from build123d import *

# Parameters (mm, degrees)
F0_R     = 5
F1_DEPTH = 2
F2_DEPTH = 2
F3_DEPTH = 2
F4_DEPTH = 2


with BuildPart() as f1:
    # F0 (on Top) → F1 (new body)
    with BuildSketch(Plane.XY):
        Circle(F0_R)
        with BuildLine():
            ThreePointArc((3.8729833462, 1), (3.9681187851, 0.5040171699), (4, 0))
            ThreePointArc((4, 0), (3.9681187851, -0.5040171699), (3.8729833462, -1))
            ThreePointArc((3.8729833462, -1), (3.5772466103, -1.789778391), (3.1224989992, -2.5))
            ThreePointArc((3.1224989992, -2.5), (2.9455449899, -2.7062455011), (2.7549954628, -2.9))
            ThreePointArc((2.7549954628, -2.9), (0, -4), (-2.7549954628, -2.9))
            ThreePointArc((-2.7549954628, -2.9), (-2.9455449899, -2.7062455011), (-3.1224989992, -2.5))
            ThreePointArc((-3.1224989992, -2.5), (-3.5772466103, -1.789778391), (-3.8729833462, -1))
            ThreePointArc((-3.8729833462, -1), (-4, 0), (-3.8729833462, 1))
            ThreePointArc((-3.8729833462, 1), (-3.5772466103, 1.789778391), (-3.1224989992, 2.5))
            ThreePointArc((-3.1224989992, 2.5), (-2.9455449899, 2.7062455011), (-2.7549954628, 2.9))
            ThreePointArc((-2.7549954628, 2.9), (0, 4), (2.7549954628, 2.9))
            ThreePointArc((2.7549954628, 2.9), (2.9455449899, 2.7062455011), (3.1224989992, 2.5))
            ThreePointArc((3.1224989992, 2.5), (3.5772466103, 1.789778391), (3.8729833462, 1))
        make_face(mode=Mode.SUBTRACT)
    extrude(amount=F1_DEPTH)

    # F0 (on Top) → F2 (join)
    with BuildSketch(Plane.XY):
        with BuildLine():
            ThreePointArc((3.8729833462, -1), (3.9681187851, -0.5040171699), (4, 0))
            ThreePointArc((4, 0), (3.9681187851, 0.5040171699), (3.8729833462, 1))
            Line((3.8729833462, 1), (-2.1040285937, 1))
            Line((-2.1040285937, 1), (-3.8729833462, 1))
            ThreePointArc((-3.8729833462, 1), (-4, 0), (-3.8729833462, -1))
            Line((-3.8729833462, -1), (-2.1040285937, -1))
            Line((-2.1040285937, -1), (3.8729833462, -1))
        make_face()
    extrude(amount=F2_DEPTH)

    # F0 (on Top) → F3 (join)
    with BuildSketch(Plane.XY):
        with BuildLine():
            Line((-2.1040285937, 2.5), (3.1224989992, 2.5))
            ThreePointArc((3.1224989992, 2.5), (2.9455449899, 2.7062455011), (2.7549954628, 2.9))
            Line((2.7549954628, 2.9), (-0.8741539787, 2.9))
            Line((-0.8741539787, 2.9), (-2.7549954628, 2.9))
            ThreePointArc((-2.7549954628, 2.9), (-2.9455449899, 2.7062455011), (-3.1224989992, 2.5))
            Line((-3.1224989992, 2.5), (-2.1040285937, 2.5))
        make_face()
    extrude(amount=F3_DEPTH)

    # F0 (on Top) → F4 (join)
    with BuildSketch(Plane.XY):
        with BuildLine():
            ThreePointArc((2.7549954628, -2.9), (2.9455449899, -2.7062455011), (3.1224989992, -2.5))
            Line((3.1224989992, -2.5), (-2.1040285937, -2.5))
            Line((-2.1040285937, -2.5), (-3.1224989992, -2.5))
            ThreePointArc((-3.1224989992, -2.5), (-2.9455449899, -2.7062455011), (-2.7549954628, -2.9))
            Line((-2.7549954628, -2.9), (-1.2980791507, -2.9))
            Line((-1.2980791507, -2.9), (2.7549954628, -2.9))
        make_face()
    extrude(amount=F4_DEPTH)


solid = f1.part
Here's how the part is built. I have some questions about the finished solid (model axes, mm). A direction names the side the tool comes from. Coordinates: 2 decimals unless noted, no trailing zeros. Write each loop counter-clockwise with the first axis right and the second up, starting at its lowest first coordinate (ties: lowest second). Pieces come first, ordered by that corner, then holes.
Item 1: If I drill on line 1 (Y direction, x = 0, z = 1.1); line 2 (Y direction, x = -3.25, z = 1.7); line 3 (Y direction, x = 1.25, z = 0.3), over which ranges is the centre line in solid material (lowest first)?
Item 2: On a 3-axis mill with a long thin cutter (end or side, diameter ignored), from which of +Z, -Z, +X, -X, +Y, -Y can I reach the whole of each face in a straight line? I mean faces 1 (the flat face through (0, 0, 0)), 2 (the flat face through (0, 2.5, 1)). Say none if no direction works.
Item 3: I want a section at D-D on x = 2. Write out the boundary of the cut face in (y, z), and give its area (3 significant figures).
Item 4: I want a section at B-B on x = 0. Write out the boundary of the cut face in (y, z), and give its area (3 significant figures).
Item 5: I want a section at C-C on y = -1.5. Write out the boundary of the cut face in (x, z).
Item 6: I want a section at A-A on z = 0.7. Write out the boundary of the cut face in (x, y) (1 decimal), and give its area (3 significant figures).
Item 7: If we mould it in two halves opening along X, with no side actions, what happens to faces 3 (the flat face through (0, 2.9, 1)), 4 (the flat face through (0, 0, 2)), 5 (the cylindrical face through (-1.08, -4.88, 0.99))? For each: +X half, -X half, draft (parallel to the pull), parting line (faces both ways), or undercut.
Findings below:
1. line 1: y = -5 to -4, -2.9 to -2.5, -1 to 1, 2.5 to 2.9, 4 to 5
1. line 2: y = -3.8 to -2.33, -1 to 1, 2.33 to 3.8
1. line 3: y = -4.84 to -3.8, -2.9 to -2.5, -1 to 1, 2.5 to 2.9, 3.8 to 4.84
2. face 1: -Z, +X, -X, +Y, -Y
2. face 2: +Z, -Z
3. outline: (-4.58, 0) - (-3.46, 0) - (-3.46, 2) - (-4.58, 2) - close; (-2.9, 0) - (-2.5, 0) - (-2.5, 2) - (-2.9, 2) - close; (-1, 0) - (1, 0) - (1, 2) - (-1, 2) - close; (2.5, 0) - (2.9, 0) - (2.9, 2) - (2.5, 2) - close; (3.46, 0) - (4.58, 0) - (4.58, 2) - (3.46, 2) - close
3. area: 10.1 mm2
4. outline: (-5, 0) - (-4, 0) - (-4, 2) - (-5, 2) - close; (-2.9, 0) - (-2.5, 0) - (-2.5, 2) - (-2.9, 2) - close; (-1, 0) - (1, 0) - (1, 2) - (-1, 2) - close; (2.5, 0) - (2.9, 0) - (2.9, 2) - (2.5, 2) - close; (4, 0) - (5, 0) - (5, 2) - (4, 2) - close
4. area: 9.60 mm2
5. outline: (-4.77, 0) - (-3.71, 0) - (-3.71, 2) - (-4.77, 2) - close; (3.71, 0) - (4.77, 0) - (4.77, 2) - (3.71, 2) - close
6. outline: circle Ø10 at (0, 0); hole (-3.9, -1) arc R4 ccw to (-3.1, -2.5) - (3.1, -2.5) arc R4 ccw to (3.9, -1) - close; hole (-3.9, 1) - (3.9, 1) arc R4 ccw to (3.1, 2.5) - (-3.1, 2.5) arc R4 ccw to start; hole (-2.8, -2.9) arc R4 ccw to (2.8, -2.9) - close; hole (-2.8, 2.9) - (2.8, 2.9) arc R4 ccw to start
6. area: 48.8 mm2
7. face 3: undercut
7. face 4: draft
7. face 5: parting line
